Job drawing, mm, ordinate dimensions from the low corner. One solid piece. Round coordinates to 2 decimals unless told otherwise and drop trailing zeros. Write each loop counter-clockwise with the first axis right and the second up, starting at its lowest first coordinate (ties: lowest second). Pieces come first, ordered by that corner, then holes. Notation, with made-up numbers: (-33, -25.5) -> (3, -25.5) arc R14 cw to (3, -1.5) -> close; hole circle Ø11 at (27, -19). An arc over 180 degrees is marked (long way). Use CSV: the item, a comma, the result in double quotes. Start each with the question number.
(1) Drop a flat-ended pin along its axis: pin 1 (2.5 mm diameter, centred on x = 4.5, y = 4.5, fed in from +Z). Give the stop position or say it passes through.
(2) Probe line 1 (X direction, y = 67.5, z = 1.1); line 2 (X direction, y = 39.5, z = 2.5); line 3 (Y direction, x = 0.75, z = 0.25). List the from-to ranges inside material, lowest first. Write a range as [from, to].
(3) Saw through at A-A (y = 67.5). Give the cut face in (x, z).
(4) Saw through at B-B (z = 2.45). Count the separate pieces of the cut face and the enclosed holes in it, plus the area to 3 significant figures.
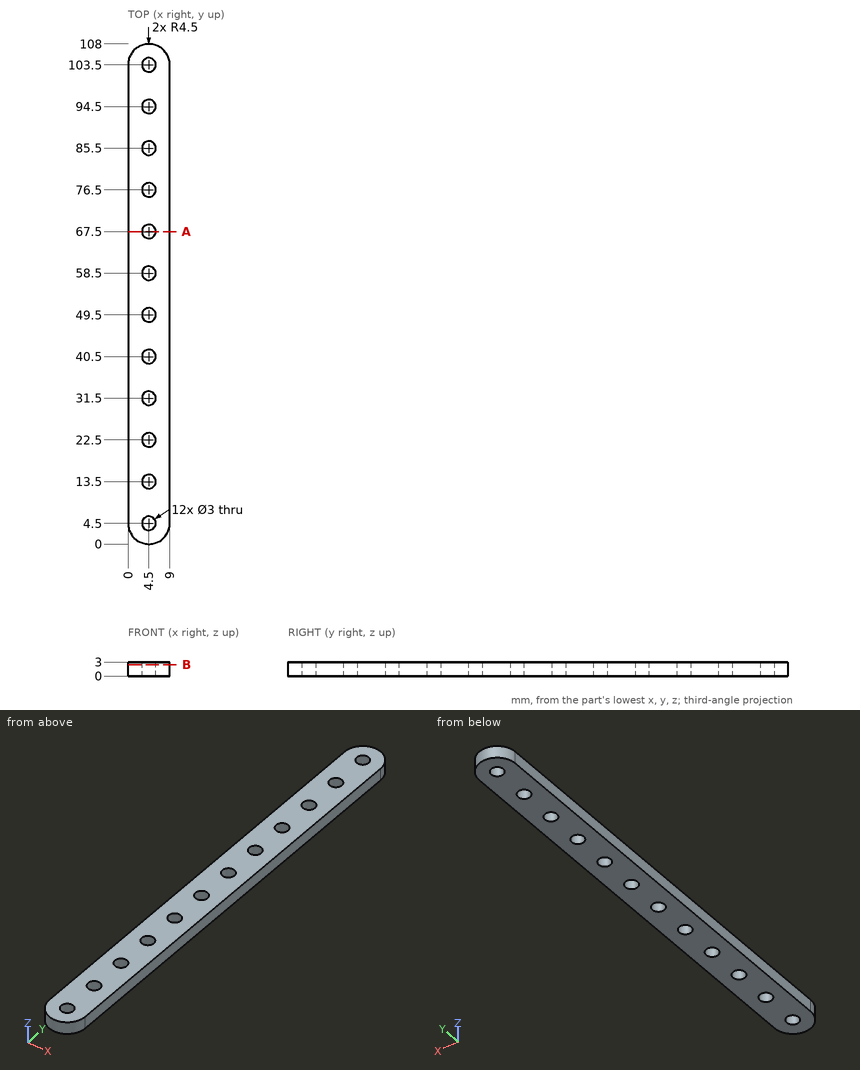
Answers:
1,pin 1,"passes through"
2,line 1,"x = [0, 3], [6, 9]"
2,line 2,"x = [0, 3.38], [5.62, 9]"
2,line 3,"y = [2.01, 105.99]"
3,outline,"(0, 0) -> (3, 0) -> (3, 3) -> (0, 3) -> close; (6, 0) -> (9, 0) -> (9, 3) -> (6, 3) -> close"
4,separate pieces,"1"
4,enclosed holes,"12"
4,area,"870 mm²"
